from build123d import *

# Parameters (mm, degrees)
PAD_DEPTH           = 46
SKETCH001_W         = 26
SKETCH001_H         = 26
POCKET_DEPTH        = 5
SKETCH002_W         = 26
SKETCH002_H         = 26
POCKET001_DEPTH     = 5
SKETCH003_W         = 26
SKETCH003_H         = 26
POCKET002_DEPTH     = 5
POCKET002_FACE2_W   = 46
POCKET002_FACE2_H   = 46
POCKET002_FACE2_W_2 = 26
POCKET002_FACE2_H_2 = 26
PAD001_DEPTH        = 13.7
PAD001_FACE1_W      = 46
PAD001_FACE1_H      = 46
PAD001_FACE1_W_2    = 26
PAD001_FACE1_H_2    = 26
PAD002_DEPTH        = 13.7
PAD002_FACE16_W     = 46
PAD002_FACE16_H     = 46
PAD002_FACE16_W_2   = 26
PAD002_FACE16_H_2   = 26
PAD003_DEPTH        = 13.7
SKETCH004_W         = 11.9
SKETCH004_H         = 42.4
POCKET003_DEPTH     = 44
SKETCH005_W         = 41
SKETCH005_H         = 36
POCKET004_DEPTH     = 5
SKETCH006_W         = 11.9
SKETCH006_H         = 42.4
POCKET005_DEPTH     = 44
SKETCH007_W         = 41
SKETCH007_H         = 36
POCKET006_DEPTH     = 5
SKETCH008_W         = 11.9
SKETCH008_H         = 42.4
POCKET007_DEPTH     = 44
SKETCH009_W         = 41
SKETCH009_H         = 36
POCKET008_DEPTH     = 5


with BuildPart() as part:
    # Sketch → Pad (new body)
    with BuildSketch(Plane.XY):
        Polygon((26.5581123827, 0), (-13.2790561914, 23), (-13.2790561914, -23), align=None)
        Polygon((23.0940107676, 0), (-11.5470053838, 20), (-11.5470053838, -20), align=None, mode=Mode.SUBTRACT)
    extrude(amount=PAD_DEPTH)

    # Sketch001 (on Face3 of Pad) → Pocket (cut)
    with BuildSketch(Plane(origin=(6.6395280957, -11.5, 0), x_dir=(0.8660254038, 0.5, 0), z_dir=(0.5, -0.8660254038, 0))):
        with Locations((0, 23)):
            Rectangle(SKETCH001_W, SKETCH001_H)
    extrude(amount=-POCKET_DEPTH, mode=Mode.SUBTRACT)

    # Sketch002 (on Face1 of Pocket) → Pocket001 (cut)
    with BuildSketch(Plane(origin=(6.6395280957, 11.5, 0), x_dir=(-0.8660254038, 0.5, 0), z_dir=(0.5, 0.8660254038, 0))):
        with Locations((0, 23)):
            Rectangle(SKETCH002_W, SKETCH002_H)
    extrude(amount=-POCKET001_DEPTH, mode=Mode.SUBTRACT)

    # Sketch003 (on Face5 of Pocket001) → Pocket002 (cut)
    with BuildSketch(Plane(origin=(-13.2790561914, 0, 0), x_dir=(0, -1, 0), z_dir=(-1, 0, 0))):
        with Locations((0, 23)):
            Rectangle(SKETCH003_W, SKETCH003_H)
    extrude(amount=-POCKET002_DEPTH, mode=Mode.SUBTRACT)

    # Pocket002 Face2 → Pad001 (add)
    with BuildSketch(Plane(origin=(6.6395280957, -11.5, 23), x_dir=(-0.8660254038, -0.5, 0), z_dir=(0.5, -0.8660254038, 0))):
        Rectangle(POCKET002_FACE2_W, POCKET002_FACE2_H)
        Rectangle(POCKET002_FACE2_W_2, POCKET002_FACE2_H_2, mode=Mode.SUBTRACT)
    extrude(amount=PAD001_DEPTH)

    # Pad001 Face1 → Pad002 (add)
    with BuildSketch(Plane(origin=(6.6395280957, 11.5, 23), x_dir=(0.8660254038, -0.5, 0), z_dir=(0.5, 0.8660254038, 0))):
        Rectangle(PAD001_FACE1_W, PAD001_FACE1_H)
        Rectangle(PAD001_FACE1_W_2, PAD001_FACE1_H_2, mode=Mode.SUBTRACT)
    extrude(amount=PAD002_DEPTH)

    # Pad002 Face16 → Pad003 (add)
    with BuildSketch(Plane(origin=(-13.2790561914, 0, 23), x_dir=(0, 1, 0), z_dir=(-1, 0, 0))):
        Rectangle(PAD002_FACE16_W, PAD002_FACE16_H)
        Rectangle(PAD002_FACE16_W_2, PAD002_FACE16_H_2, mode=Mode.SUBTRACT)
    extrude(amount=PAD003_DEPTH)

    # Sketch004 (on Face4 of Pad003) → Pocket003 (cut)
    with BuildSketch(Plane(origin=(19.918584287, -11.5, 0), x_dir=(0.5, 0.8660254038, 0), z_dir=(0.8660254038, -0.5, 0))):
        with Locations((19.2290561914, 23)):
            Rectangle(SKETCH004_W, SKETCH004_H)
    extrude(amount=-POCKET003_DEPTH, mode=Mode.SUBTRACT)

    # Sketch005 (on Face14 of Pocket003) → Pocket004 (cut)
    with BuildSketch(Plane(origin=(13.4895280957, 23.3645480318, 0), x_dir=(-0.8660254038, 0.5, 0), z_dir=(0.5, 0.8660254038, 0))):
        with Locations((-2.5, 23)):
            Rectangle(SKETCH005_W, SKETCH005_H)
    extrude(amount=-POCKET004_DEPTH, mode=Mode.SUBTRACT)

    # Sketch006 (on Face41 of Pocket004) → Pocket005 (cut)
    with BuildSketch(Plane(origin=(0, 23, 0), x_dir=(-1, 0, 0), z_dir=(0, 1, 0))):
        with Locations((19.2290561914, 23)):
            Rectangle(SKETCH006_W, SKETCH006_H)
    extrude(amount=-POCKET005_DEPTH, mode=Mode.SUBTRACT)

    # Sketch007 (on Face40 of Pocket005) → Pocket006 (cut)
    with BuildSketch(Plane(origin=(-26.9790561914, 0, 0), x_dir=(0, -1, 0), z_dir=(-1, 0, 0))):
        with Locations((-2.5, 23)):
            Rectangle(SKETCH007_W, SKETCH007_H)
    extrude(amount=-POCKET006_DEPTH, mode=Mode.SUBTRACT)

    # Sketch008 (on Face8 of Pocket006) → Pocket007 (cut)
    with BuildSketch(Plane(origin=(-19.918584287, -11.5, 0), x_dir=(0.5, -0.8660254038, 0), z_dir=(-0.8660254038, -0.5, 0))):
        with Locations((19.2290561914, 23)):
            Rectangle(SKETCH008_W, SKETCH008_H)
    extrude(amount=-POCKET007_DEPTH, mode=Mode.SUBTRACT)

    # Sketch009 (on Face7 of Pocket007) → Pocket008 (cut)
    with BuildSketch(Plane(origin=(13.4895280957, -23.3645480318, 0), x_dir=(0.8660254038, 0.5, 0), z_dir=(0.5, -0.8660254038, 0))):
        with Locations((-2.5, 23)):
            Rectangle(SKETCH009_W, SKETCH009_H)
    extrude(amount=-POCKET008_DEPTH, mode=Mode.SUBTRACT)


solid = part.part
Read the model definition and answer for the solid it produces. Units are mm, in the model's axes. A direction names the side the tool comes from. Give positions to 0.01 mm unless a question says otherwise; leave off trailing zeros. Loops run counter-clockwise (first coordinate to the right, second up) from the corner with the lowest first, then second, coordinate; pieces in that order, holes last. Notation, with made-up numbers: (36.5, 36) - (41.5, 36) arc R28 ccw to (41.5, 65) - close; hole circle Ø5 at (-8, 21). An arc over 180 degrees is marked (long way). Answer as CSV lines item,"result". Start each with the question number.
1) Straight lines are drawn through the part: L1, parallel to Z at x = 22, y = 17.5; L2, parallel to Y at x = 22, z = 42; L3, parallel to Z at x = -2, y = 23.5. For each, find the intervals that lie inside material, in ascending order. Write a range as from..to.
2) Find section B-B (z = 38). Write down the section's boundary in (x, y), then the cut area to 3 significant figures.
3) Which of the six approach directions +Z, -Z, +X, -X, +Y, -Y give full straight-line access (tool end or side, diameter ignored) to faces 4 (the face through (-19, -21, 23)), 5 (the face through (11, 16, 1.8)), 6 (the face through (30.7, 7.17, 1.42))?
4) Find section A-A (z = 22). State how many separate pieces and enclosed holes the cut face has, then the cut area to 3 significant figures.
5) Determine the mould class of faces 1 (the face through (-2.54, 31.6, 22.75)), 2 (the face through (6, 11, 36)), 3 (the face through (-9.9, 28.85, 23.32)) for opening direction Z: released by +Z, released by -Z, zero draft, split by the parting line, or undercut.
6) Each of these flat-tipped pins is pushed along its axis until it touches: pin 1 Ø6 at (y, z) = (0, 27.5) entering from -X; pin 2 Ø6 at (x, z) = (-17.5, 15) entering from +Y; pin 3 Ø7 at (x, z) = (-18, 14.5) entering from -Y; pin 4 Ø1.5 at (x, y) = (6, 8) entering from -Z. Where does it stop, or does it pass through?
7) Find section D-D (y = -30.5). Write down the section's boundary in (x, z).
Findings below:
1,L1,"0..5, 41..46"
1,L2,"-18.45..-16.37, -2.63..-0.63, 0.63..2.63, 16.37..18.45"
1,L3,"0..1.8, 44.2..46"
2,outline,"(-26.98, -23) - (-13.28, -23) - (24.83, -1) - (30.78, -11.31) - (28.18, -12.81) - (29.08, -14.36) - (33.41, -11.86) - (26.56, 0) - (-11.55, 22) - (-5.6, 32.31) - (-3, 30.81) - (-2.1, 32.36) - (-6.43, 34.86) - (-13.28, 23) - (-13.28, -21) - (-25.18, -21) - (-25.18, -18) - (-26.98, -18) - close; hole (-11.55, -20) - (23.09, 0) - (-11.55, 20) - close"
2,area,"322 mm^2"
3,face 4,"+Y"
3,face 5,"none"
3,face 6,"+Z, -Z, +X"
4,separate pieces,"3"
4,enclosed holes,"0"
4,area,"187 mm^2"
5,face 1,"undercut"
5,face 2,"undercut"
5,face 3,"zero draft"
6,pin 1,"x = 17.9"
6,pin 2,"y = -21"
6,pin 3,"y = -23"
6,pin 4,"through"
7,outline,"(-8.95, 0) - (1.13, 0) - (1.13, 5) - (-2.47, 5) - (-2.47, 1.8) - (-8.95, 1.8) - close; (-8.95, 44.2) - (-2.47, 44.2) - (-2.47, 41) - (1.13, 41) - (1.13, 46) - (-8.95, 46) - close"
